```python
from build123d import *

# Parameters (mm, degrees)
SKETCH1_W           = 75
SKETCH1_H           = 12.7
SKETCH1_R           = 2
BOSS_EXTRUDE1_DEPTH = 12.7
SKETCH2_R           = 5
CUT_EXTRUDE1_DEPTH  = 12.7


with BuildPart() as part:
    # Sketch1 → Boss-Extrude1 (new body)
    with BuildSketch(Plane(origin=(0, 0, 0), x_dir=(1, 0, 0), z_dir=(0, 1, 0))):
        Rectangle(SKETCH1_W, SKETCH1_H)
        with Locations((-32, 0)):
            Circle(SKETCH1_R, mode=Mode.SUBTRACT)
        with Locations((-22, 0)):
            Circle(SKETCH1_R, mode=Mode.SUBTRACT)
        with Locations((22, 0)):
            Circle(SKETCH1_R, mode=Mode.SUBTRACT)
        with Locations((32, 0)):
            Circle(SKETCH1_R, mode=Mode.SUBTRACT)
    extrude(amount=BOSS_EXTRUDE1_DEPTH)

    # Sketch2 → Cut-Extrude1 (cut)
    with BuildSketch(Plane.XY.offset(6.35)):
        with Locations((-3.5, 6.35)):
            Circle(SKETCH2_R)
        with Locations((4.005771179, 6.35)):
            Circle(SKETCH2_R)
    extrude(amount=-CUT_EXTRUDE1_DEPTH, mode=Mode.SUBTRACT)


solid = part.part
```
Source: CAD feature listing. Evaluate the final solid. Frame: model axes, mm. Give positions to 0.01 mm unless a question says otherwise; leave off trailing zeros. Order: outer loops, then holes, each group sorted by start corner. A loop starts at its lowest first (then second) coordinate and runs counter-clockwise, first axis right, second up. Notation, with made-up numbers: (40.25, 6.25) -> (47.25, 6.25) arc R27 cw to (47.25, 42.25) -> close; hole circle Ø7 at (8, 61.5). An arc over 180 degrees is marked (long way). Use a Markdown table: item, result.
Q1. Material intervals for line 1 (X direction, y = 7, z = 0); line 2 (Y direction, x = -3.5, z = 1); line 3 (X direction, y = 3.25, z = 0), sorted ascending. Write a range as [from, to].
A:
| item | result |
|---|---|
| line 1 | [-37.5, -34], [-30, -24], [-20, -8.46], [8.96, 20], [24, 30], [34, 37.5] |
| line 2 | [0, 1.35], [11.35, 12.7] |
| line 3 | [-37.5, -34], [-30, -24], [-20, -7.42], [7.93, 20], [24, 30], [34, 37.5] |
Q2. Section A-A (y = 6.35). Return the cut outline in (x, z).
A:
| item | result |
|---|---|
| outline | (-37.5, -6.35) -> (-8.5, -6.35) -> (-8.5, 6.35) -> (-37.5, 6.35) -> close; (9.01, -6.35) -> (37.5, -6.35) -> (37.5, 6.35) -> (9.01, 6.35) -> close; hole circle Ø4 at (-32, 0); hole circle Ø4 at (-22, 0); hole circle Ø4 at (22, 0); hole circle Ø4 at (32, 0) |
Q3. Section C-C (z = 0). Return the cut outline in (x, y), and give its area (3 significant figures).
A:
| item | result |
|---|---|
| outline | (-37.5, 0) -> (-34, 0) -> (-34, 12.7) -> (-37.5, 12.7) -> close; (-30, 0) -> (-24, 0) -> (-24, 12.7) -> (-30, 12.7) -> close; (-20, 0) -> (20, 0) -> (20, 12.7) -> (-20, 12.7) -> close; (24, 0) -> (30, 0) -> (30, 12.7) -> (24, 12.7) -> close; (34, 0) -> (37.5, 0) -> (37.5, 12.7) -> (34, 12.7) -> close; hole (0.25, 3.05) arc R5 ccw (long way) to (0.25, 9.65) arc R5 ccw (long way) to start |
| area | 604 mm^2 |
Q4. Section B-B (x = 22). Return the cut outline in (y, z).
A:
| item | result |
|---|---|
| outline | (0, -6.35) -> (12.7, -6.35) -> (12.7, -2) -> (0, -2) -> close; (0, 2) -> (12.7, 2) -> (12.7, 6.35) -> (0, 6.35) -> close |
Q5. Section D-D (x = -3.5). Return the cut outline in (y, z).
A:
| item | result |
|---|---|
| outline | (0, -6.35) -> (1.35, -6.35) -> (1.35, 6.35) -> (0, 6.35) -> close; (11.35, -6.35) -> (12.7, -6.35) -> (12.7, 6.35) -> (11.35, 6.35) -> close |
Q6. Pull-direction query (X, two-part tool) for faces 1 (the face through (20.4, 6.3, 1.2)), 2 (the face through (-0.5, 2, 6.35)), 3 (the face through (-37.5, 6, 0)); classes: +X half, -X half, draft (parallel to the pull), parting line (faces both ways), or undercut.
A:
| item | result |
|---|---|
| face 1 | undercut |
| face 2 | draft |
| face 3 | -X half |
